Design review of the part shown in the three views and the two pictorial views. Dimensions are in mm from the part's minimum x, y and z. Round coordinates to 2 decimals unless told otherwise and drop trailing zeros. Order: outer loops, then holes, each group sorted by start corner. A loop starts at its lowest first (then second) coordinate and runs counter-clockwise, first axis right, second up.
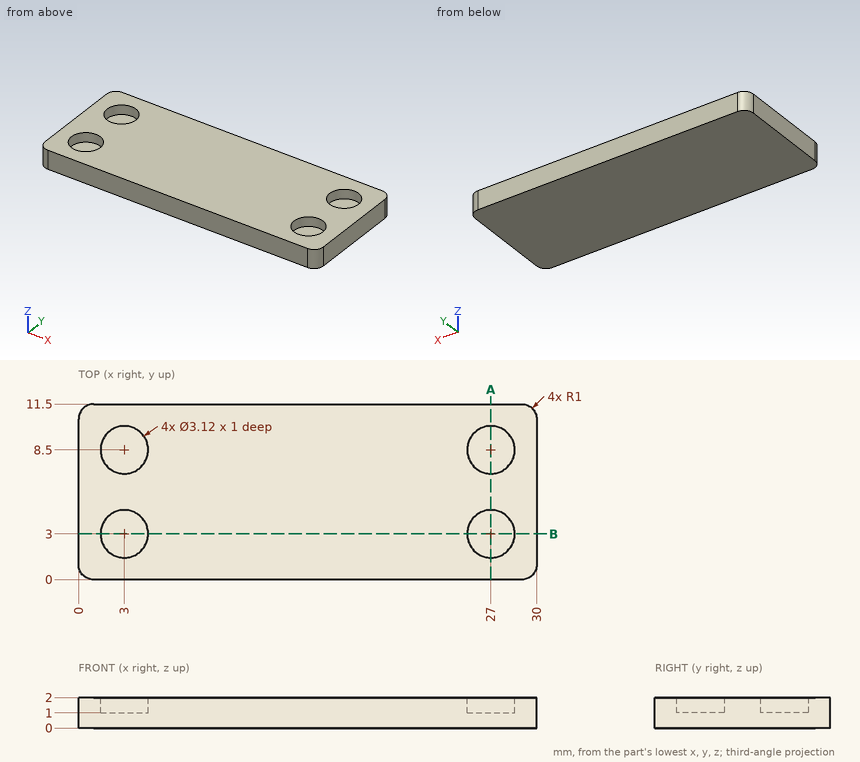
(1) Consider section B-B (y = 3). Write out the cut boundary in (x, z).
Data:
outline: (0, 0) - (30, 0) - (30, 2) - (28.56, 2) - (28.56, 1) - (25.44, 1) - (25.44, 2) - (4.56, 2) - (4.56, 1) - (1.44, 1) - (1.44, 2) - (0, 2) - close
(2) Insertion check: pin 1 (0.9 mm diameter, centred on x = 3, y = 2.5, fed in from +Z). The pin has a flat end and moves straight along its axis. Give the tip position at first contact, or say it passes through.
Data:
pin 1: stops at z = 1
(3) Consider section A-A (x = 27). Write out the cut boundary in (y, z).
Data:
outline: (0, 0) - (11.5, 0) - (11.5, 2) - (10.06, 2) - (10.06, 1) - (6.94, 1) - (6.94, 2) - (4.56, 2) - (4.56, 1) - (1.44, 1) - (1.44, 2) - (0, 2) - close
(4) To check wall thickness, follow probe 1 along Y at (x, z) = (3, 1.6); probe 2 along X at (y, z) = (8.5, 1.2); probe 3 along X at (y, z) = (7.5, 1.15) (1 decimal). State the ranges of each line that lie inside material, in increasing order.
Data:
probe 1: y = 0 to 1.44, 4.56 to 6.94, 10.06 to 11.5
probe 2: x = 0 to 1.44, 4.56 to 25.44, 28.56 to 30
probe 3: x = 0 to 1.8, 4.2 to 25.8, 28.2 to 30
